Could you check a few things on this model? Use its own coordinates, in mm. Coordinates: 2 decimals unless noted, no trailing zeros. Write each loop counter-clockwise with the first axis right and the second up, starting at its lowest first coordinate (ties: lowest second). Pieces come first, ordered by that corner, then holes.
Autodesk Inventor part; units mm, degrees
ref_plane "YZ Plane" through (0, 0, 0) normal (1, 0, 0) x (0, 1, 0)
ref_plane "XZ Plane" through (0, 0, 0) normal (0, 1, 0) x (-1, 0, 0)
ref_plane "XY Plane" through (0, 0, 0) normal (0, 0, 1) x (1, 0, 0)
sketch "Sketch1" plane through (0, 0, 0) normal (0, 0, 1) x (1, 0, 0)
  line L0 (0, 0) -> (38.1, 0)
  line L1 (38.1, 0) -> (38.1, 253.0348)
  arc A0 (38.1, 507.0348) -> (38.1, 253.0348) centre (666.75, 380.0348) ccw
  line L2 (38.1, 507.0348) -> (38.1, 608.6348)
  line L3 (38.1, 608.6348) -> (0, 608.6348)
  line L4 (0, 608.6348) -> (0, 0)
  circle A1 centre (31.75, 151.4348) radius 3.3655
  circle A2 centre (31.75, 34.671) radius 3.3655
  circle A3 centre (12.7, 12.7) radius 3.3655
  circle A4 centre (12.7, 342.9) radius 3.3655
  circle A5 centre (12.7, 595.9348) radius 3.3655
  circle A6 centre (31.75, 12.7) radius 3.3655
  circle A7 centre (31.75, 253.0348) radius 3.3655
  circle A8 centre (31.75, 507.0348) radius 3.3655
  circle A9 centre (31.75, 595.9348) radius 3.3655
  line L5 (0, 557.8348) -> (0, 608.6348)
  line L6 (0, 50.8) -> (0, 0)
  line L7 (12.7, 342.9) -> (0, 304.3174) construction
  line L8 (0, 317.5) -> (0, 368.3)
  line L9 (0, 129.921) -> (12.7, 129.921) construction
  circle A10 centre (12.7, 129.921) radius 3.3655
  circle A11 centre (12.7, 174.371) radius 3.3655
  line L10 (9.3413, 197.482) -> (9.3413, 204.213)
  line L11 (16.0611, 204.488) -> (16.0611, 197.3435)
  arc A12 (16.0611, 204.488) -> (9.3413, 204.213) centre (12.6956, 204.488) ccw
  arc A13 (9.3413, 197.482) -> (16.0611, 197.3435) centre (12.6974, 197.231) ccw
  circle A14 centre (12.7, 217.188) radius 3.3655
  dimension "d0" = 38.1
  dimension "d2" = 101.6
  dimension "d4" = 457.2
  dimension "d5" = 101.6
  dimension "d6" = 666.75
  dimension "d7" = 641.35
  dimension "d9" = 116.7638
  dimension "d10" = 6.35
  dimension "d11" = 6.35
  dimension "d13" = 12.7
  dimension "d14" = 12.7
  dimension "d16" = 12.7
  dimension "d17" = 342.9
  dimension "d19" = 12.7
  dimension "d20" = 12.7
  dimension "d22" = 6.35
  dimension "d24" = 6.35
  dimension "d25" = 6.731
  dimension "d26" = 6.35
  dimension "hole" = 6.731
  dimension "d28" = 6.35
  dimension "d45" = 12.7
  dimension "d47" = 12.7
  dimension "d54" = 6.731
  dimension "d55" = 3.3655
  dimension "d56" = 3.3655
  dimension "d58" = 6.731
  dimension "d59" = 12.7
  dimension "d68" = 18.22
  dimension "d69" = 90
  dimension "d70" = 90
  dimension "d71" = 22.0389
  dimension "d72" = 28.7587
  dimension "d73" = 478.7138
  dimension "d74" = 6.35
  dimension "d75" = 6.35
  dimension "d76" = 595.9348
  dimension "d77" = 404.1468
  dimension "d78" = 411.2913
  dimension "d79" = 25.4
  dimension "d80" = 25.4
  dimension "d81" = 434.2638
  dimension "d82" = 50.8
  dimension "d83" = 240.3348
  dimension "d84" = 291.1348
  dimension "d85" = 557.8348
extrude "Extrusion2" add sketch "Sketch1" along normal blind 25.4
fillet "Fillet1" radius 6.096 2 edges at (0, 184.15, 25.4) (0, 488.4674, 25.4)
equation "\"d25\" = hole"
equation "\"BendRadius\" = Thickness"
equation "\"BendReliefWidth\" = Thickness"
equation "\"BendReliefDepth\" = 0.5 * Thickness"
equation "\"CornerReliefSize\" = 4 * Thickness"
equation "\"MinimumRemnant\" = 2 * Thickness"
equation "\"TransitionRadius\" = BendRadius"
equation "\"JacobiRadiusSize\" = BendRadius"
equation "\"GapSize\" = Thickness"
equation "\"d29\" = BendRadius"
equation "\"d32\" = BendRadius"
equation "\"d38\" = BendRadius"
equation "\"d60\" = BendRadius"
properties part number "Claw - Arm - Top (R) Bottom"
Item 1: I want a section at A-A, the plane z = 7. Count the separate pieces of the cut face and the enclosed holes in it, then the cut area to 3 significant figures.
Item 2: I want a section at B-B, the plane y = 490. List the corners of the cut face in (x, z) for me.
Item 3: If I drill on line 1 along X through (y, z) = (218, 5.25); line 2 along Z through (x, y) = (6, 384.5); line 3 along X through (y, z) = (207, 1), over which ranges is the centre line in solid material (lowest first)?
Item 4: I want a section at C-C, the plane y = 419.5. List the corners of the cut face in (x, z) for me, then the cut area to 3 significant figures.
Item 5: If we mould it in two halves opening along Y, with no side actions, what happens to faces 1 (the flat face through (19, 0, 13)), 2 (the flat face through (0, 309, 10)), 3 (the cylindrical face through (25.402, 378.245, 12.522))? For each: released by +Y, released by -Y, zero draft, split by the parting line, or undercut.
Item 6: Will this pin go through, and if not, where does the flat tip stop? pin 1 Ø2 at (y, z) = (199.5, 6.5) entering from -X.
Taken from the geometry:
1. separate pieces: 1
1. enclosed holes: 13
1. area: 20,500 mm2
2. outline: (0, 0) - (34.9, 0) - (34.9, 25.4) - (6.1, 25.4) arc R6.1 ccw to (0, 19.3) - close
3. line 1: x = 0 to 9.43, 15.97 to 38.1
3. line 2: z = 0 to 25.4
3. line 3: x = 0 to 10.46, 14.94 to 38.1
4. outline: (0, 0) - (26.62, 0) - (26.62, 25.4) - (6.1, 25.4) arc R6.1 ccw to (0, 19.3) - close
4. area: 668 mm2
5. face 1: released by -Y
5. face 2: zero draft
5. face 3: undercut
6. pin 1: stops at x = 0
